Autodesk Inventor part; units mm, degrees
ref_plane "ANBAU_XY" through (0, 0, 0) normal (0, 1, 0) x (1, 0, 0)
ref_plane "ANBAU_YZ" through (0, 0, 0) normal (1, 0, 0) x (0, 0, -1)
ref_plane "ANBAU_ZX" through (0, 0, 0) normal (0, 0, -1) x (0, 1, 0)
sketch "Sketch_1" plane through (0, 0, 0) normal (0, 0, 1) x (1, 0, 0)
  line L0 (0, -20) -> (0, 4)
  line L1 (0, 1.134) -> (1.5, 2)
  line L2 (1.5, 2) -> (1.5, 3.7679)
  line L3 (1.5, 3.7679) -> (1.7321, 4)
  line L4 (1.7321, 4) -> (3.1, 4)
  line L5 (3.1, 4) -> (3.5, 3.6)
  line L6 (3.5, 3.6) -> (3.5, 0.1)
  line L7 (3.5, 0.1) -> (3.4, 0)
  line L8 (3.4, 0) -> (2.05, 0)
  line L9 (2.05, 0) -> (2, -0.6)
  line L10 (2, -0.6) -> (2, -19.5705)
  line L11 (2, -19.5705) -> (1.5705, -20)
  line L12 (1.5705, -20) -> (0, -20)
  line L13 (0, -20) -> (0, 1.134)
revolve "Revolution1" add sketch "Sketch_1" angle 360 about axis through (0, -20, 0) along (0, -1, 0)
thread "Thread1"
sketch "Sketch_2" plane through (0, 4, 0) normal (0, 1, 0) x (1, 0, 0)
  line L0 (-1.5, -0.866) -> (0, -1.7321)
  line L1 (0, -1.7321) -> (1.5, -0.866)
  line L2 (1.5, -0.866) -> (1.5, 0.866)
  line L3 (1.5, 0.866) -> (0, 1.7321)
  line L4 (0, 1.7321) -> (-1.5, 0.866)
  line L5 (-1.5, 0.866) -> (-1.5, -0.866)
extrude "Extrusion1" cut sketch "Sketch_2" against normal blind 2
ref_plane "ANBAU_XY" through (0, 0, 0) normal (0, 1, 0) x (1, 0, 0)
ref_plane "ANBAU_YZ" through (0, 0, 0) normal (1, 0, 0) x (0, 0, -1)
ref_plane "ANBAU_ZX" through (0, 0, 0) normal (0, 0, -1) x (0, 1, 0)
ref_plane "Schraube_XY" through (0, 0, 0) normal (0, 1, 0) x (1, 0, 0)
ref_plane "Schraube_YZ" through (0, 0, 0) normal (1, 0, 0) x (0, 0, -1)
ref_plane "Schraube_ZX" through (0, 0, 0) normal (0, 0, -1) x (0, 1, 0)
ref_plane "insert_XY" through (0, 0, 0) normal (0, 1, 0) x (1, 0, 0)
ref_plane "insert_YZ" through (0, 0, 0) normal (1, 0, 0) x (0, 0, -1)
ref_plane "insert_ZX" through (0, 0, 0) normal (0, 0, -1) x (0, 1, 0)
ref_plane "schrauben_punkt_XY" through (0, -20, 0) normal (0, 1, 0) x (1, 0, 0)
ref_plane "schrauben_punkt_YZ" through (0, -20, 0) normal (1, 0, 0) x (0, 0, -1)
ref_plane "schrauben_punkt_ZX" through (0, -20, 0) normal (0, 0, -1) x (0, 1, 0)
properties part number "DIN-912 - M4x20(F)"
Source: CAD feature listing. Evaluate the final solid. Frame: model axes, mm. A direction names the side the tool comes from. Coordinates: 2 decimals unless noted, no trailing zeros. Loops run counter-clockwise (first coordinate to the right, second up) from the corner with the lowest first, then second, coordinate; pieces in that order, holes last. Notation, with made-up numbers: M -28,42 L -18,42 A18 cw -18,48 Z; hole C 31,52.5 d8. An arc over 180 degrees is marked long. Use a Markdown table: item, result. Add a question column.
Q1. Section query A-A, the plane y = -4.25. Return loops of the section in (x, z), and give its area (3 significant figures).
Q2. Access query for faces 1 (the flat face through (0.761, 3.014, -1.293)), 2 (the flat face through (1.334, 4, -1.334)). Directions: +Z, -Z, +X, -X, +Y, -Y. A direction counts if a zero-diameter tool reaches every point of the face in a straight line with its end or side. Return the directions, or none.
Q3. First-contact query: pin 1 (0.9 mm diameter, centred on x = 0, z = -1, fed in from +Y); pin 2 (1.5 mm diameter, centred on x = -2, y = -5.5, fed in from +Z); pin 3 (2 mm diameter, centred on y = -6.5, z = 2, fed in from -X). Flat tips, straight axial feed; report the tip coordinate or a pass-through.
Q4. Material intervals for L1, parallel to X at y = -4.5, z = -1; L2, parallel to Y at x = 1.5, z = 1.5, sorted ascending.
Q5. Draft query along Z for faces 3 (the cylindrical face through (0, -10, -2)), 4 (the flat face through (0, 0, -2.2)), 5 (the flat face through (0.74, 3.014, 1.305)). Return one class per face: pulls with the +Z half, pulls with the -Z half, needs draft (parallel to the pull), parting line crosses it, or undercut.
Result:
| question | item | result |
|---|---|---|
| 1 | outline | C 0,0 d4 |
| 1 | area | 12.6 mm2 |
| 2 | face 1 | +Y |
| 2 | face 2 | +Z, -Z, +X, -X, +Y |
| 3 | pin 1 | stops at y = 1.97 |
| 3 | pin 2 | stops at z = 1.56 |
| 3 | pin 3 | stops at x = -1.73 |
| 4 | L1 | x = -1.73 to 1.73 |
| 4 | L2 | y = 0 to 4 |
| 5 | face 3 | parting line crosses it |
| 5 | face 4 | needs draft |
| 5 | face 5 | undercut |
